```python
from build123d import *

# Parameters (mm, degrees)
F0_W = 3.9116
F0_H = 19.0754
F3_D = 7.62


with BuildPart() as f1:
    # F0 (on Front) → F1 (revolve)
    with BuildSketch(Plane.XZ):
        Polygon((-42.7736, 0), (0, 0), (0, 9.0424), (-25.6286, 9.0424), (-42.7736, 9.0424), align=None)
        Polygon((-25.6286, 9.0424), (0, 9.0424), (0, 16.8656), (-11.7348, 16.8656), (-15.6464, 16.8656), (-25.6286, 16.8656), align=None)
        with Locations((-13.6906, 26.4033)):
            Rectangle(F0_W, F0_H)
    revolve(axis=Axis((-21.3868, 0, 0), (-1, 0, 0)))

    # F3 (through all)
    with Locations(Plane.YZ):
        with Locations((0, 0)):
            Hole(F3_D / 2)


solid = f1.part
```
CAD build for the part. Positions are in the model's coordinates, mm. A direction names the side the tool comes from. Coordinates: 2 decimals unless noted, no trailing zeros. Order: outer loops, then holes, each group sorted by start corner. A loop starts at its lowest first (then second) coordinate and runs counter-clockwise, first axis right, second up. Notation, with made-up numbers: (85.25, 4.25) - (129.25, 4.25) arc R26 ccw to (129.25, 39.25) - close; hole circle Ø6 at (49, 3.5). An arc over 180 degrees is marked (long way). Use a Markdown table: item, result. Add a question column.
(1) Which spindle directions (+Z, -Z, +X, -X, +Y, -Y) get a long thin tool onto all of the face, cutting with end or side? Do faces 1 (the face through (-11.735, -15.5, -7.5)), 2 (the face through (0, 0, 4)), 3 (the face through (-20.71, 16.72, -2.2)). Say none if no direction does.
(2) Flat gauge pins, fed straight in: pin 1 (3 mm diameter, centred on x = -12.5, y = -8.5, fed in from -Z); pin 2 (6 mm diameter, centred on y = 23, z = -26.5, fed in from +X); pin 3 (8 mm diameter, centred on y = 10.5, z = -15, fed in from -X). Where does each tip first touch, or does it go through?
(3) Drill centre lines: line 1 along Y through (x, z) = (-22, -1.5); line 2 along Y through (x, z) = (-34.5, 1); line 3 along X through (y, z) = (-17, 28). Where is each one in solid material? Low to high. Write a range as [from, to].
(4) Saw through at D-D (y = -14.5). Give the cut face in (x, z).
(5) Saw through at A-A (y = 0). Give the cut face in (x, z).
(6) Saw through at C-C (x = -30). Give the cut face in (y, z).
(7) Pull direction Z, two halves, no side cores. Call faces 4 (the face through (-25.629, -7, 7)), 5 (the face through (-5.95, 16.72, -2.2)), 6 (the face through (-21.69, 0.83, -3.72)): +Z half, -Z half, draft (parallel to the pull), parting line (faces both ways), or undercut.
Solved:
| question | item | result |
|---|---|---|
| 1 | face 1 | +X |
| 1 | face 2 | +Z, -Z, +X, +Y, -Y |
| 1 | face 3 | -X |
| 2 | pin 1 | stops at z = -35.25 |
| 2 | pin 2 | stops at x = -11.73 |
| 2 | pin 3 | stops at x = -25.63 |
| 3 | line 1 | y = [-16.8, -3.5], [3.5, 16.8] |
| 3 | line 2 | y = [-8.99, -3.68], [3.68, 8.99] |
| 3 | line 3 | x = [-15.65, -11.73] |
| 4 | outline | (-25.63, -8.61) - (-15.65, -8.61) - (-15.65, -32.89) - (-11.73, -32.89) - (-11.73, -8.61) - (0, -8.61) - (0, 8.61) - (-11.73, 8.61) - (-11.73, 32.89) - (-15.65, 32.89) - (-15.65, 8.61) - (-25.63, 8.61) - close |
| 5 | outline | (-42.77, -9.04) - (-25.63, -9.04) - (-25.63, -16.87) - (-15.65, -16.87) - (-15.65, -35.94) - (-11.73, -35.94) - (-11.73, -16.87) - (0, -16.87) - (0, -3.81) - (-42.77, -3.81) - close; (-42.77, 3.81) - (0, 3.81) - (0, 16.87) - (-11.73, 16.87) - (-11.73, 35.94) - (-15.65, 35.94) - (-15.65, 16.87) - (-25.63, 16.87) - (-25.63, 9.04) - (-42.77, 9.04) - close |
| 6 | outline | circle Ø18.08 at (0, 0); hole circle Ø7.62 at (0, 0) |
| 7 | face 4 | draft |
| 7 | face 5 | parting line |
| 7 | face 6 | undercut |
